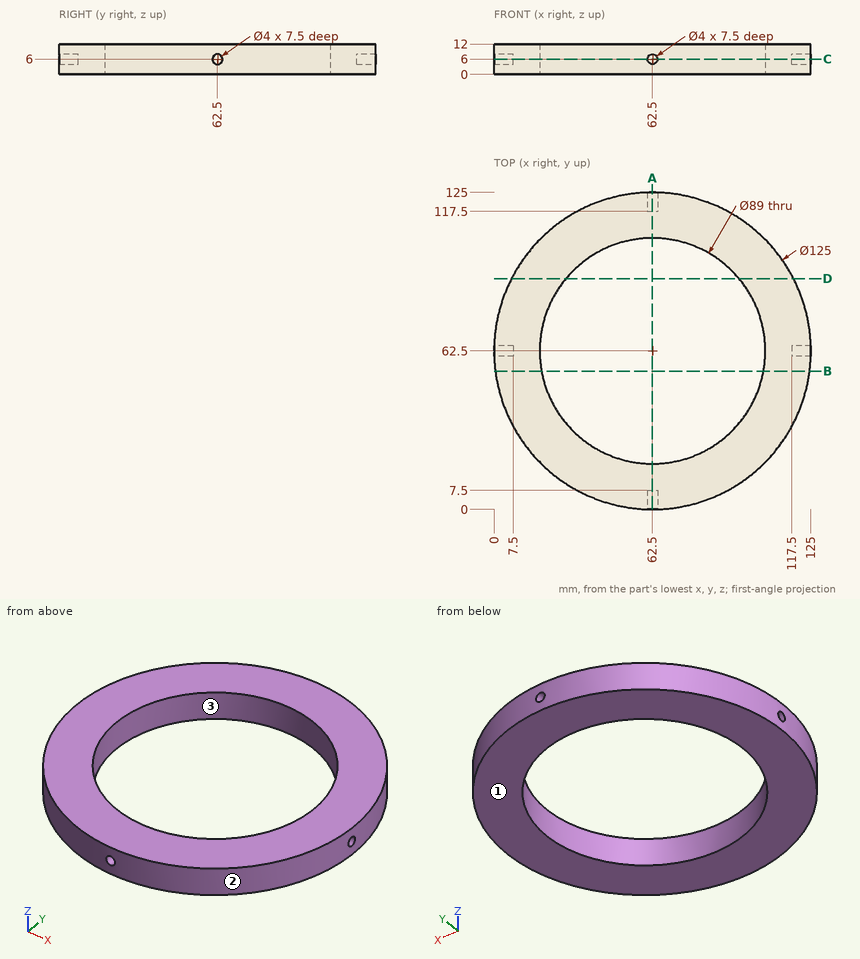
Here's the drawing with two shaded views (mm, measured from the low corner). I have some questions. Round coordinates to 2 decimals unless told otherwise and drop trailing zeros. Order: outer loops, then holes, each group sorted by start corner. A loop starts at its lowest first (then second) coordinate and runs counter-clockwise, first axis right, second up. Notation, with made-up numbers: (26, 61.25) -> (51, 61.25) arc R18 ccw to (51, 83.25) -> close; hole circle Ø8 at (36, 43.5). An arc over 180 degrees is marked (long way). Write each question's results on one line, items separated by ' | '. Start each with the question number.
Item 1: Thinking about a two-plate mould opening in X: for the marked faces 1, 2 and 3, which applies, +X half, -X half, draft (parallel to the pull), parting line (faces both ways), or undercut?
Item 2: If we section it at D-D, the plane y = 91: Write out the boundary of the cut face in (x, z), then the cut area to 3 significant figures.
Item 3: If we section it at A-A, the plane x = 62.5: Write out the boundary of the cut face in (y, z), then the cut area to 3 significant figures.
Item 4: If we section it at B-B, the plane y = 54.5: Write out the boundary of the cut face in (x, z) (3 decimals), then the cut area to 3 significant figures.
Item 5: If we section it at C-C, the plane z = 6: Write out the boundary of the cut face in (x, y), then the cut area to 3 significant figures.
Item 6: Will these pins go through, and if not, where does the flat tip stop? pin 1 (6 mm diameter, centred on x = 91.5, z = 8.5, fed in from +Y); pin 2 (1.5 mm diameter, centred on y = 100.5, z = 7, fed in from +X); pin 3 (3.5 mm diameter, centred on x = 62.5, z = 6, fed in from +Y).
Item 7: Please list where these lines run through material, in increasing order: L1, parallel to Y at x = 68, z = 5.5; L2, parallel to Z at x = 3, y = 62; L3, parallel to Y at x = 120.25, z = 6.
Results:
1) face 1: draft | face 2: parting line | face 3: undercut
2) outline: (6.88, 0) -> (28.32, 0) -> (28.32, 12) -> (6.88, 12) -> close; (96.68, 0) -> (118.12, 0) -> (118.12, 12) -> (96.68, 12) -> close | area: 515 mm2
3) outline: (0, 0) -> (18, 0) -> (18, 12) -> (0, 12) -> (0, 8) -> (7.5, 8) -> (7.5, 4) -> (0, 4) -> close; (107, 0) -> (125, 0) -> (125, 4) -> (117.5, 4) -> (117.5, 8) -> (125, 8) -> (125, 12) -> (107, 12) -> close | area: 372 mm2
4) outline: (0.514, 0) -> (18.725, 0) -> (18.725, 12) -> (0.514, 12) -> close; (106.275, 0) -> (124.486, 0) -> (124.486, 12) -> (106.275, 12) -> close | area: 437 mm2
5) outline: (0.03, 60.5) arc R62.5 ccw to (60.5, 0.03) -> (60.5, 7.5) -> (64.5, 7.5) -> (64.5, 0.03) arc R62.5 ccw to (124.97, 60.5) -> (117.5, 60.5) -> (117.5, 64.5) -> (124.97, 64.5) arc R62.5 ccw to (64.5, 124.97) -> (64.5, 117.5) -> (60.5, 117.5) -> (60.5, 124.97) arc R62.5 ccw to (0.03, 64.5) -> (7.5, 64.5) -> (7.5, 60.5) -> close; hole circle Ø89 at (62.5, 62.5) | area: 5,930 mm2
6) pin 1: stops at y = 119.34 | pin 2: stops at x = 112.69 | pin 3: stops at y = 117.5
7) L1: y = 0.24 to 18.34, 106.66 to 124.76 | L2: z = 0 to 4.06, 7.94 to 12 | L3: y = 38.6 to 60.5, 64.5 to 86.4
